from build123d import *

# Parameters (mm, degrees)
F1_DEPTH = 30
F2_R     = 10
F3_DEPTH = 4
F4_W     = 24
F4_H     = 24
F4_W_2   = 20
F4_H_2   = 20
F5_DEPTH = 43.5
F6_W     = 20
F6_H     = 14.353989
F7_DEPTH = 28.1


with BuildPart() as f1:
    # F0 (on Front) → F1 (new body)
    with BuildSketch(Plane.XZ):
        Polygon((-27.424138, -47.5), (27.424138, -47.5), (54.848276, 0), (27.424138, 47.5), (-27.424138, 47.5), (-54.848276, 0), align=None)
        Polygon((50.229473, 0), (25.114737, -43.5), (-25.114737, -43.5), (-50.229473, 0), (-25.114737, 43.5), (25.114737, 43.5), align=None, mode=Mode.SUBTRACT)
    extrude(amount=F1_DEPTH)

    # F2 (on face) → F3 (cut, through all)
    with BuildSketch(Plane(origin=(0, 0, -47.5), x_dir=(1, 0, 0), z_dir=(0, 0, -1))):
        with Locations((0, 15)):
            Circle(F2_R)
    extrude(amount=-F3_DEPTH, mode=Mode.SUBTRACT)

    # F4 (on face) → F5 (join)
    with BuildSketch(Plane.XY.offset(-43.5)):
        with Locations((0, -15)):
            Rectangle(F4_W, F4_H)
        with Locations((0, -15)):
            Rectangle(F4_W_2, F4_H_2, mode=Mode.SUBTRACT)
    extrude(amount=F5_DEPTH)

    # F6 (on face) → F7 (cut)
    with BuildSketch(Plane.XZ.offset(27)):
        with Locations((0, -7.176994)):
            Rectangle(F6_W, F6_H)
    extrude(amount=-F7_DEPTH, mode=Mode.SUBTRACT)


solid = f1.part
Part model, mm, in its own coordinate system. A direction names the side the tool comes from. Coordinates: 2 decimals unless noted, no trailing zeros. Order: outer loops, then holes, each group sorted by start corner. A loop starts at its lowest first (then second) coordinate and runs counter-clockwise, first axis right, second up.
(1) Slice it at B-B, the plane z = -29. Write the cut outline in (x, y).
Check sheet entries:
outline: (-38.11, -30) - (-33.49, -30) - (-33.49, 0) - (-38.11, 0) - close; (-12, -27) - (12, -27) - (12, -3) - (-12, -3) - close; (33.49, -30) - (38.11, -30) - (38.11, 0) - (33.49, 0) - close; hole (-10, -25) - (10, -25) - (10, -5) - (-10, -5) - close
(2) Slice it at C-C, the plane z = 26. Write the cut outline in (x, y).
Check sheet entries:
outline: (-39.84, -30) - (-35.22, -30) - (-35.22, 0) - (-39.84, 0) - close; (35.22, -30) - (39.84, -30) - (39.84, 0) - (35.22, 0) - close
(3) Slice it at A-A, the plane x = 17. Write the cut outline in (y, z).
Check sheet entries:
outline: (-30, -47.5) - (0, -47.5) - (0, -43.5) - (-30, -43.5) - close; (-30, 43.5) - (0, 43.5) - (0, 47.5) - (-30, 47.5) - close
(4) Pin check, flat tips, straight feed: pin 1 Ø10 at (x, z) = (-1.5, -35.5) entering from +Y; pin 2 Ø2 at (x, y) = (40, -13.5) entering from +Z; pin 3 Ø5 at (x, y) = (42, -11.5) entering from -Z. Stop position of each tip, or through.
Check sheet entries:
pin 1: stops at y = -3
pin 2: stops at z = 27.45
pin 3: stops at z = -26.58
(5) Probe L1, parallel to Y at x = 0, z = -45; L2, parallel to Z at x = -21, y = -4; L3, parallel to X at y = -15.5, z = -8. List the from-to ranges inside material, lowest first.
Check sheet entries:
L1: y = -30 to -25, -5 to 0
L2: z = -47.5 to -43.5, 43.5 to 47.5
L3: x = -50.23 to -45.61, -12 to -10, 10 to 12, 45.61 to 50.23
(6) Pull direction Y, two halves, no side cores. Call faces 1 (the face through (-40.944, -14.79, 24.082)), 2 (the face through (-10, -15, -22)), 3 (the face through (0, -3, -27)): pulls with the +Y half, pulls with the -Y half, needs draft (parallel to the pull), parting line crosses it, or undercut.
Check sheet entries:
face 1: needs draft
face 2: undercut
face 3: pulls with the +Y half
(7) Slice it at D-D, the plane y = -12. Write the cut outline in (x, z).
Check sheet entries:
outline: (-54.85, 0) - (-27.42, -47.5) - (-9.54, -47.5) - (-9.54, -43.5) - (-10, -43.5) - (-10, 0) - (-12, 0) - (-12, -43.5) - (-25.11, -43.5) - (-50.23, 0) - (-25.11, 43.5) - (25.11, 43.5) - (50.23, 0) - (25.11, -43.5) - (12, -43.5) - (12, 0) - (10, 0) - (10, -43.5) - (9.54, -43.5) - (9.54, -47.5) - (27.42, -47.5) - (54.85, 0) - (27.42, 47.5) - (-27.42, 47.5) - close
(8) Tool access for faces 4 (the face through (-12, -15, -22)), 5 (the face through (0, -27, -27)), 6 (the face through (40.4, 0, -17.4)), 7 (the face through (0, -25, -29)), 8 (the face through (0, -15, 47.5)): list every direction of +Z, -Z, +X, -X, +Y, -Y with a clear straight run to the whole face (end or side of a thin tool).
Check sheet entries:
face 4: +Y, -Y
face 5: -Y
face 6: +Z, -Z, +X, -X, +Y
face 7: none
face 8: +Z, +X, -X, +Y, -Y
